from build123d import *

# Parameters (mm, degrees)
SKETCH1_R          = 28.25
BASE_EXTRUDE_DEPTH = 7


with BuildPart() as part:
    # Sketch1 → Base-Extrude (new body)
    with BuildSketch(Plane.XY):
        with BuildLine():
            ThreePointArc((34.37992312, 29.034821961), (-45, 0), (34.37992312, -29.034821961))
            ThreePointArc((34.37992312, -29.034821961), (50.650379443, -17.946188292), (70.309608401, -16.850623426))
            ThreePointArc((70.309608401, -16.850623426), (91.25, 0), (70.309608401, 16.850623426))
            ThreePointArc((70.309608401, 16.850623426), (50.650379443, 17.946188292), (34.37992312, 29.034821961))
        make_face()
        Circle(SKETCH1_R, mode=Mode.SUBTRACT)
    extrude(amount=BASE_EXTRUDE_DEPTH)


solid = part.part
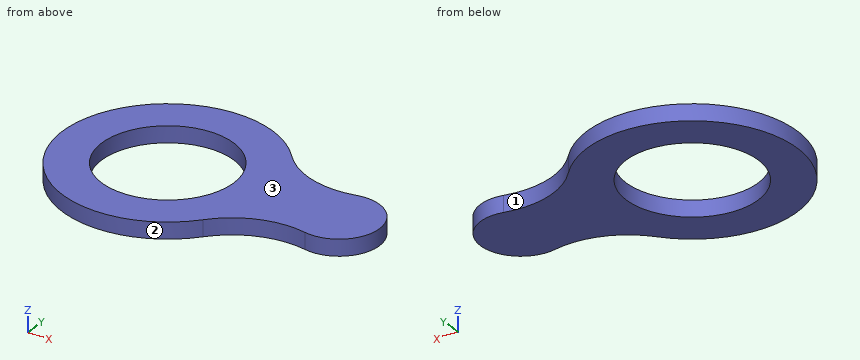
Can you work these out from the model? Positions are in its coordinate system, mm. Face numbers are marked on the shaded views. Give positions to 0.01 mm unless a question says otherwise; leave off trailing zeros. Order: outer loops, then holes, each group sorted by start corner. A loop starts at its lowest first (then second) coordinate and runs counter-clockwise, first axis right, second up. Notation, with made-up numbers: M 61,9 L 79,9 A24 ccw 79,23 Z; hole C 3.25,77 d7. An arc over 180 degrees is marked long. One line per item, written item: value.
Item 1: If we mould it in two halves opening along X, with no side actions, what happens to the marked faces 1, 2 and 3? For each: pulls with the +X half, pulls with the -X half, needs draft (parallel to the pull), parting line crosses it, or undercut.
Verdict:
face 1: undercut
face 2: parting line crosses it
face 3: needs draft
Item 2: If we section it at C-C on z = 4.75: Write out the boundary of the cut face in (x, y).
Verdict:
outline: M 34.38,-29.03 A36.74 cw 70.31,-16.85 A17.25 ccw long 70.31,16.85 A36.74 cw 34.38,29.03 A45 ccw long Z; hole C 0,0 d56.5
Item 3: If we section it at D-D on x = 74: Write out the boundary of the cut face in (y, z), and give its area (4 significant figures).
Verdict:
outline: M -17.25,0 L 17.25,0 L 17.25,7 L -17.25,7 Z
area: 241.5 mm2
Item 4: If we section it at A-A on y = 0: Write out the boundary of the cut face in (x, z), and give its area (3 significant figures).
Verdict:
outline: M -45,0 L -28.25,0 L -28.25,7 L -45,7 Z; M 28.25,0 L 91.25,0 L 91.25,7 L 28.25,7 Z
area: 558 mm2
Item 5: If we section it at B-B on x = 0: Write out the boundary of the cut face in (y, z).
Verdict:
outline: M -45,0 L -28.25,0 L -28.25,7 L -45,7 Z; M 28.25,0 L 45,0 L 45,7 L 28.25,7 Z
Item 6: For pin 1 (5 mm diameter, centred on x = 35.5, y = -34, fed in from -Z); pin 2 (3 mm diameter, centred on x = 20.5, y = -27.5, fed in from -Z), each with a flat end and sliding along its axis, tell me the tip position at first contact or that it passes through.
Verdict:
pin 1: through
pin 2: z = 0
Item 7: Please list where these lines run through material, in increasing order: line 1 (Y direction, x = 0, z = 4.25); line 2 (Y direction, x = 14, z = 4); line 3 (X direction, y = 10.5, z = 4.75).
Verdict:
line 1: -45 to -28.25, 28.25 to 45
line 2: -42.77 to -24.54, 24.54 to 42.77
line 3: -43.76 to -26.23, 26.23 to 87.69
